Work out the finished part from the listing and answer in its coordinate system (mm). A direction names the side the tool comes from. Coordinates: 2 decimals unless noted, no trailing zeros. Write each loop counter-clockwise with the first axis right and the second up, starting at its lowest first coordinate (ties: lowest second). Pieces come first, ordered by that corner, then holes. Notation, with made-up numbers: (2, 87) - (17, 87) arc R25 ccw to (17, 125) - close; hole circle Ø7 at (69, -36). An arc over 180 degrees is marked (long way). Use CSV: the item, a comma, the result in double quotes. Start each with the question number.
Autodesk Inventor part; units mm, degrees
sketch "Skizze1" plane through (0, 0, 0) normal (0, 0, 1) x (1, 0, 0)
  line L0 (-57, 28) -> (57, 28)
  line L1 (57, 28) -> (57, -28)
  line L2 (57, -28) -> (-57, -28)
  line L3 (-57, -28) -> (-57, 28)
  line L4 (0, -39.2) -> (0, 39.2)
  line L5 (-79.8, 0) -> (79.8, 0)
  circle A0 centre (-47.5, 0) radius 1.5
  circle A1 centre (47.5, 0) radius 1.5
  circle A2 centre (-50, -12.5) radius 4
  point P0 (0, 0)
  dimension "d0" = 114
  dimension "d1" = 56
  dimension "d2" = 3
  dimension "d3" = 47.5
  dimension "d4" = 8
  dimension "d5" = 40.5
  dimension "d6" = 7
extrude "Extrusion1" add sketch "Skizze1" along normal mid plane 11 contours L0 L4 L5 A0 L3 | L0 L1 L5 A1 L4 | L5 A0 L4 L2 L3 | L5 A1 L1 L2 L4
sketch "Skizze2" plane through (0, 0, -5.5) normal (0, 0, -1) x (-1, 0, 0)
  line L0 (57, -28) -> (57, 28)
  line L1 (-57, 28) -> (-57, -28)
  line L2 (55, -28) -> (55, 28)
  line L3 (-55, 28) -> (-55, -28)
  line L4 (55, -28) -> (-55, -28)
  line L5 (-55, 28) -> (55, 28)
  line L6 (-57, 28) -> (57, 28)
  point P0 (0, 0)
  dimension "d9" = 2
  dimension "d10" = 2
extrude "Extrusion2" cut sketch "Skizze2" against normal blind 8
fillet "Rundung1" radius 2 2 edges at (-57, 0, 5.5) (57, 0, 5.5)
fillet "Rundung2" radius 2 2 edges at (-55, 0, 2.5) (55, 0, 2.5)
properties part number "KarosserieDachTeil4"
Item 1: A cutting plane is placed at D-D (x = 0). Determine the outline of the cut face in (y, z).
Item 2: A cutting plane is placed at B-B (x = -47.5). Determine the outline of the cut face in (y, z), then the cut area to 3 significant figures.
Item 3: Determine the mould class of faces 1 (the face through (56.4, 0.39, 4.93)), 2 (the face through (-49, 0, 4)), 3 (the face through (-1, 0, 5.5)) for opening direction X: +X half, -X half, draft (parallel to the pull), parting line (faces both ways), or undercut.
Item 4: Which of the six approach directions +Z, -Z, +X, -X, +Y, -Y give full straight-line access (tool end or side, diameter ignored) to faces 4 (the face through (57, 0, -1)), 5 (the face through (-55, 0, -3))?
Item 5: A cutting plane is placed at A-A (z = -1.25). Determine the outline of the cut face in (x, y), then the cut area to 3 significant figures.
Item 6: Each of these flat-tipped pins is pushed along its axis until it touches: pin 1 (4 mm diameter, centred on x = 20.5, y = 0, fed in from -Z); pin 2 (7 mm diameter, centred on x = -50, y = -12.5, fed in from +Z). Where does it stop, or does it pass through?
Item 7: A cutting plane is placed at C-C (y = 24.5). Determine the outline of the cut face in (x, z), then the cut area to 3 significant figures.
Item 8: Straight lines are drawn through the part: probe 1 along X at (y, z) = (19, -3); probe 2 along Y at (x, z) = (-50, 4.8); probe 3 along X at (y, z) = (-12.5, 3.75). For each, find the intervals that lie inside material, in ascending order. Write a range as [from, to].
Calculated:
1,outline,"(-28, 2.5) - (28, 2.5) - (28, 5.5) - (-28, 5.5) - close"
2,outline,"(-28, 2.5) - (-15.62, 2.5) - (-15.62, 5.5) - (-28, 5.5) - close; (-9.38, 2.5) - (-1.5, 2.5) - (-1.5, 5.5) - (-9.38, 5.5) - close; (1.5, 2.5) - (28, 2.5) - (28, 5.5) - (1.5, 5.5) - close"
2,area,"140 mm²"
3,face 1,"+X half"
3,face 2,"undercut"
3,face 3,"draft"
4,face 4,"+Z, -Z, +X, +Y, -Y"
4,face 5,"-Z, +Y, -Y"
5,outline,"(-57, -28) - (-55, -28) - (-55, 28) - (-57, 28) - close; (55, -28) - (57, -28) - (57, 28) - (55, 28) - close"
5,area,"224 mm²"
6,pin 1,"stops at z = 2.5"
6,pin 2,"passes through"
7,outline,"(-57, -5.5) - (-55, -5.5) - (-55, 0.5) arc R2 cw to (-53, 2.5) - (53, 2.5) arc R2 cw to (55, 0.5) - (55, -5.5) - (57, -5.5) - (57, 3.5) arc R2 ccw to (55, 5.5) - (-55, 5.5) arc R2 ccw to (-57, 3.5) - close"
7,area,"374 mm²"
8,probe 1,"x = [-57, -55], [55, 57]"
8,probe 2,"y = [-28, -16.5], [-8.5, 28]"
8,probe 3,"x = [-56.98, -54], [-46, 56.98]"
